Verification items for this drawing (mm, ordinates from the low corner). Give positions to 0.01 mm unless a question says otherwise; leave off trailing zeros. Loops run counter-clockwise (first coordinate to the right, second up) from the corner with the lowest first, then second, coordinate; pieces in that order, holes last. Notation, with made-up numbers: (4.5, 66) -> (45.5, 66) arc R30 ccw to (45.5, 101) -> close; hole circle Ø5 at (6.25, -34.75). An arc over 180 degrees is marked (long way). Write each question's results on one line, items separated by ' | '. Start each with the question number.
Item 1: Cross-section at D-D on x = 16.75. Enter the section's corners in (y, z) (1 decimal), then the cut area to 3 significant figures.
Item 2: Cross-section at A-A on x = 2.25. Enter the section's corners in (y, z) (1 decimal), then the cut area to 3 significant figures.
Item 3: Cross-section at C-C on y = 31.5. Enter the section's corners in (x, z).
Item 4: Gauge pin test, flat ends, axial feed: pin 1 Ø10 at (x, y) = (12.5, 8.5) entering from -Z; pin 2 Ø5 at (x, y) = (18, 32) entering from -Z; pin 3 Ø1.5 at (x, y) = (17, 18) entering from -Z. Record the tip position at first contact, or that the pin passes through.
Item 5: Scan lines: line 1 along Y through (x, z) = (23.75, 21.5) (1 decimal); line 2 along Y through (x, z) = (3.25, 11) (1 decimal); line 3 along Y through (x, z) = (7, 31) (1 decimal). Record each from-to range of solid material in increasing order.
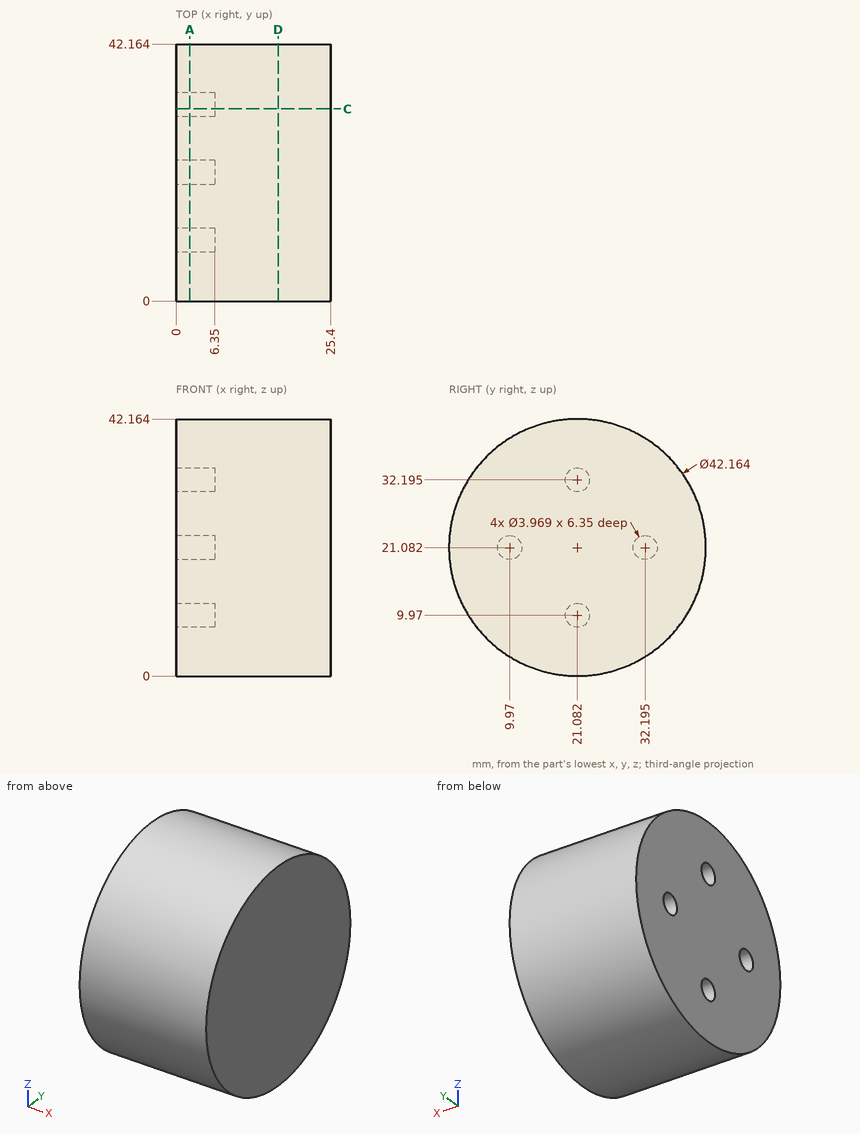
Answer sheet:
1) outline: circle Ø42.2 at (21.1, 21.1) | area: 1,400 mm²
2) outline: circle Ø42.2 at (21.1, 21.1); hole circle Ø4 at (10, 21.1); hole circle Ø4 at (21.1, 10); hole circle Ø4 at (21.1, 32.2); hole circle Ø4 at (32.2, 21.1) | area: 1,350 mm²
3) outline: (0, 2.75) -> (25.4, 2.75) -> (25.4, 39.41) -> (0, 39.41) -> (0, 22.94) -> (6.35, 22.94) -> (6.35, 19.22) -> (0, 19.22) -> close
4) pin 1: stops at z = 1.41 | pin 2: stops at z = 1.75 | pin 3: stops at z = 0.13
5) line 1: y = 0 to 42.2 | line 2: y = 2.6 to 19.4, 22.8 to 39.6 | line 3: y = 2.5 to 39.7
